Model file for the job. Use its own axes, mm. A direction names the side the tool comes from. Round coordinates to 2 decimals unless told otherwise and drop trailing zeros. Write each loop counter-clockwise with the first axis right and the second up, starting at its lowest first coordinate (ties: lowest second). Pieces come first, ordered by that corner, then holes. Notation, with made-up numbers: (54, 51) - (109, 51) arc R35 cw to (109, 87) - close; hole circle Ø8 at (88.25, 46). An arc over 180 degrees is marked (long way). One line per item, written item: value.
Autodesk Inventor part; units mm, degrees
ref_plane "YZ Plane" through (0, 0, 0) normal (1, 0, 0) x (0, 1, 0)
ref_plane "XZ Plane" through (0, 0, 0) normal (0, 1, 0) x (-1, 0, 0)
ref_plane "XY Plane" through (0, 0, 0) normal (0, 0, 1) x (1, 0, 0)
sketch "Sketch1" plane through (0, 0, 0) normal (0, 0, 1) x (1, 0, 0)
  line L0 (-8.9346, 3.531) -> (-24.9346, 3.531)
  line L1 (-24.9346, 3.531) -> (-24.9346, 45.531)
  line L2 (17.0654, 45.531) -> (17.0654, 3.531)
  line L3 (17.0654, 3.531) -> (1.0654, 3.531)
  line L4 (-8.9346, -0.469) -> (1.0654, -0.469)
  line L5 (-8.9346, 3.531) -> (-8.9346, -0.469)
  line L6 (1.0654, 3.531) -> (1.0654, -0.469)
  line L7 (17.0654, 45.531) -> (3.6736, 45.531)
  line L8 (-24.9346, 45.531) -> (-11.5428, 45.531)
  arc A0 (-11.5428, 45.531) -> (3.6736, 45.531) centre (-3.9346, 49.8809) ccw
  point P0 (0, 0)
extrude "Extrusion4" add sketch "Sketch1" against normal blind 5
sketch "Sketch2" plane through (17.0654, 3.531, 0) normal (1, 0, 0) x (0, 0, -1)
  line L0 (0, 42) -> (5, 42)
  line L1 (0, 42) -> (0, 39.5)
  line L2 (0, 37.5859) -> (0, 42)
  line L3 (0, 39.5) -> (5, 39.5)
  line L4 (5, 42) -> (5, 37.5859)
  circle A0 centre (2.5, 39.5) radius 1.5
  point P0 (0, -3.531)
hole "Hole1" at (17.0654, 43.031, -2.5) direction (-1, 0, 0) diameter 3 depth 5 tip angle 118
sketch "Sketch3" plane through (-24.9346, 3.531, 0) normal (-1, 0, 0) x (0, 0, 1)
  circle A0 centre (-2.5, 39.5) radius 1.5
  circle A1 centre (-2.5, 39.5) radius 1.5
  point P0 (0, -3.531)
hole "Hole2" at (-24.9346, 43.031, -2.5) direction (1, 0, 0) diameter 3 depth 5 tip angle 118
properties part number "suport continuare seringa" material "Gold"
1. Mould opens along Z. For faces 6 (the face through (-4, -0.469, -2)), 7 (the face through (-19.19, 42.8, -2.38)), 8 (the face through (-4, 23, -5)), 9 (the face through (-22.4, 44.5, -2.8)) say: released by +Z, released by -Z, zero draft, split by the parting line, or undercut.
Report:
face 6: zero draft
face 7: undercut
face 8: released by -Z
face 9: undercut
2. Band-saw the part on B-B on x = 7. Write the cut outline in (y, z), plus the area to 3 significant figures.
Report:
outline: (3.53, -5) - (45.53, -5) - (45.53, 0) - (3.53, 0) - close
area: 210 mm²
3. Tool access for faces 1 (the face through (14.5, 44.5, -2.2)), 2 (the face through (9, 3.531, -2)), 3 (the face through (-17, 3.531, -2)), 4 (the face through (-18, 45.531, -2)), 5 (the face through (-24.935, 24, -2)): list every direction of +Z, -Z, +X, -X, +Y, -Y with a clear straight run to the whole face (end or side of a thin tool).
Report:
face 1: +X
face 2: +Z, -Z, +X, -Y
face 3: +Z, -Z, -X, -Y
face 4: +Z, -Z, +X, -X, +Y
face 5: +Z, -Z, -X, +Y, -Y
4. Band-saw the part on C-C on x = -3. Write the cut outline in (y, z), plus the area to 3 significant figures.
Report:
outline: (-0.47, -5) - (41.17, -5) - (41.17, 0) - (-0.47, 0) - close
area: 208 mm²
5. Wall check: probe 1 along Y at (x, z) = (-23.65, -2.5); probe 2 along Y at (x, z) = (9, -0.5); probe 3 along X at (y, z) = (44, -2.75). Give the ranges that are in metal, low to high. Write a range as [from, to].
Report:
probe 1: [3.53, 41.53], [44.53, 45.53]
probe 2: [3.53, 45.53]
probe 3: [-19.63, -10.43], [2.56, 11.77]
6. Band-saw the part on A-A on z = -4.5. Write the cut outline in (x, y), plus the area to 3 significant figures.
Report:
outline: (-24.93, 3.53) - (-8.93, 3.53) - (-8.93, -0.47) - (1.07, -0.47) - (1.07, 3.53) - (17.07, 3.53) - (17.07, 45.53) - (3.67, 45.53) arc R8.76 cw to (-11.54, 45.53) - (-24.93, 45.53) - close
area: 1,760 mm²
7. Drop a flat-ended pin along its axis: pin 1 (1.5 mm diameter, centred on x = 11, z = -2, fed in from -Y). Give the stop position or say it passes through.
Report:
pin 1: y = 3.53
